The drawing under review shows one solid part. Ordinate dimensions are in mm from its lowest x, y, z. A direction names the side the tool comes from. Coordinates: 2 decimals unless noted, no trailing zeros. Loops run counter-clockwise (first coordinate to the right, second up) from the corner with the lowest first, then second, coordinate; pieces in that order, holes last. Notation, with made-up numbers: (80.5, 82.25) - (117.5, 82.25) arc R16 ccw to (117.5, 113.25) - close; hole circle Ø8 at (85.25, 85.5). An arc over 180 degrees is marked (long way). Answer as a JSON object with one key per item and string values. Group by question number.
Item 1: We need section A-A (y = 5). Give the boundary of the cut face in (x, z).
Item 2: Mouldability with a two-part tool opening along X and no side actions: class the marked faces 4, 5 and 6 as released by +X, released by -X, zero draft, split by the parting line, or undercut.
Item 3: Clearance check with flat-ended pins moving along their axes: pin 1 (3 mm diameter, centred on x = 9, z = 14.5, fed in from +Y); pin 2 (2 mm diameter, centred on x = 4.5, y = 8.5, fed in from +Z); pin 3 (3 mm diameter, centred on x = 3, z = 12.5, fed in from +Y). State where each tip first meets the part, or that it passes through.
Item 4: We need section C-C (z = 5). Give the boundary of the cut face in (x, y).
Item 5: To check wall thickness, follow line 1 (Z direction, x = 2.5, y = 8.25); line 2 (Y direction, x = 6.25, z = 1.5) (1 decimal); line 3 (Y direction, x = 5, z = 8.5). State the ranges of each line that lie inside material, in increasing order.
Item 6: Tool access review of the marked faces 1, 2 and 3: name each direction out of +Z, -Z, +X, -X, +Y, -Y from which nothing blocks a thin tool from reaching the whole face with its end or side.
Item 7: We need section B-B (z = 7.5). Give the boundary of the cut face in (x, y), then the cut area to 3 significant figures.
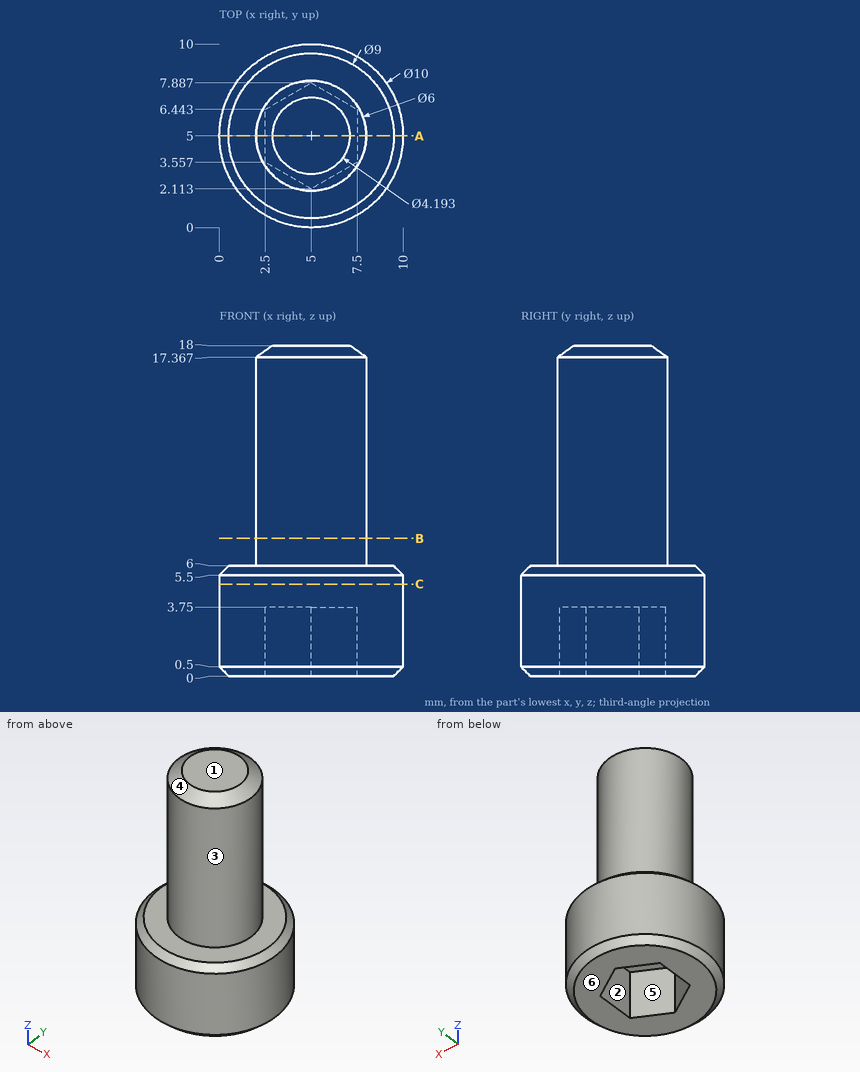
Check sheet entries:
{
 "1": {"outline": "(0, 0.5) - (0.5, 0) - (2.5, 0) - (2.5, 3.75) - (7.5, 3.75) - (7.5, 0) - (9.5, 0) - (10, 0.5) - (10, 5.5) - (9.5, 6) - (8, 6) - (8, 17.37) - (7.1, 18) - (2.9, 18) - (2, 17.37) - (2, 6) - (0.5, 6) - (0, 5.5) - close"},
 "2": {"face 4": "split by the parting line", "face 5": "undercut", "face 6": "zero draft"},
 "3": {"pin 1": "stops at y = 6.66", "pin 2": "stops at z = 17.69", "pin 3": "stops at y = 7.96"},
 "4": {"outline": "circle Ø10 at (5, 5)"},
 "5": {"line 1": "z = 0 to 6", "line 2": "y = 0.2 to 2.8, 7.2 to 9.8", "line 3": "y = 2 to 8"},
 "6": {"face 1": "+Z, +X, -X, +Y, -Y", "face 2": "-Z", "face 3": "+Z"},
 "7": {"outline": "circle Ø6 at (5, 5)", "area": "28.3 mm2"}
}
